from build123d import *

# Parameters (mm, degrees)
SCHIZZO1_R                        = 1.5
ESTRUSIONE_ESTRUSIONE1_DEPTH      = 4.5
ESTRUSIONE_ESTRUSIONE1_DEPTH_BACK = 4.5
SCHIZZO2_W                        = 32
SCHIZZO2_H                        = 3
SCHIZZO2_W_2                      = 10
TAGLIO_ESTRUSIONE1_DEPTH          = 12.277661417
TAGLIO_ESTRUSIONE1_DEPTH_BACK     = 23.284267349
TAGLIO_ESTRUSIONE3_DEPTH          = 3.5
RACCORDO1_R                       = 5
RACCORDO2_R                       = 5
RACCORDO3_R                       = 2.5
RACCORDO4_R                       = 2.5


with BuildPart() as part:
    # Schizzo1 → Estrusione-Estrusione1 (new body, two sides)
    with BuildSketch(Plane.XY) as estrusione_estrusione1_sk:
        with BuildLine():
            ThreePointArc((9.895231175, 3), (-10.34, 0), (9.895231175, -3))
            Line((9.895231175, -3), (35, -3))
            ThreePointArc((35, -3), (38, 0), (35, 3))
            Line((35, 3), (9.895231175, 3))
        make_face()
        Circle(SCHIZZO1_R, mode=Mode.SUBTRACT)
        with Locations((35, 0)):
            Circle(SCHIZZO1_R, mode=Mode.SUBTRACT)
    extrude(amount=ESTRUSIONE_ESTRUSIONE1_DEPTH)
    extrude(estrusione_estrusione1_sk.sketch, amount=-ESTRUSIONE_ESTRUSIONE1_DEPTH_BACK)

    # Schizzo2 → Taglio-Estrusione1 (cut, two sides)
    with BuildSketch(Plane(origin=(0, -3, 0), x_dir=(-1, 0, 0), z_dir=(0, -1, 0))) as taglio_estrusione1_sk:
        with Locations((-5.66, 0)):
            Rectangle(SCHIZZO2_W, SCHIZZO2_H)
        with Locations((-33, 0)):
            Rectangle(SCHIZZO2_W_2, SCHIZZO2_H)
    extrude(amount=TAGLIO_ESTRUSIONE1_DEPTH, mode=Mode.SUBTRACT)
    extrude(taglio_estrusione1_sk.sketch, amount=-TAGLIO_ESTRUSIONE1_DEPTH_BACK, mode=Mode.SUBTRACT)

    # Schizzo18 → Taglio-Estrusione3 (cut)
    with BuildSketch(Plane(origin=(0, 0, -4.5), x_dir=(-1, 0, 0), z_dir=(0, 0, -1))):
        with BuildLine():
            Line((-9.895231175, 3), (-5.58530214, 3))
            ThreePointArc((-5.58530214, 3), (6.34, 0), (-5.58530214, -3))
            Line((-5.58530214, -3), (-9.895231175, -3))
            ThreePointArc((-9.895231175, -3), (10.34, 0), (-9.895231175, 3))
        make_face()
    extrude(amount=-TAGLIO_ESTRUSIONE3_DEPTH, mode=Mode.SUBTRACT)

    # Raccordo1
    raccordo1_edges = [part.edges().sort_by_distance(p)[0] for p in [
        (9.895231175, 3, 3),
    ]]
    fillet(raccordo1_edges, radius=RACCORDO1_R)

    # Raccordo2
    raccordo2_edges = [part.edges().sort_by_distance(p)[0] for p in [
        (9.895231175, -3, 3),
    ]]
    fillet(raccordo2_edges, radius=RACCORDO2_R)

    # Raccordo3
    raccordo3_edges = [part.edges().sort_by_distance(p)[0] for p in [
        (5.58530214, 3, -3),
    ]]
    fillet(raccordo3_edges, radius=RACCORDO3_R)

    # Raccordo4
    raccordo4_edges = [part.edges().sort_by_distance(p)[0] for p in [
        (5.58530214, -3, -3),
    ]]
    fillet(raccordo4_edges, radius=RACCORDO4_R)


solid = part.part
Model file for the job. Use its own axes, mm. A direction names the side the tool comes from. Round coordinates to 2 decimals unless told otherwise and drop trailing zeros. Loops run counter-clockwise (first coordinate to the right, second up) from the corner with the lowest first, then second, coordinate; pieces in that order, holes last. Notation, with made-up numbers: M 65,85.25 L 78,85.25 A23 cw 78,96.25 Z; hole C 41.25,-25 d1. An arc over 180 degrees is marked long. One line per question, with ' | ' between items.
1) Mould opens along Z. For faces 5 (the cylindrical face through (5.82, -3.255, -2.979)), 6 (the flat face through (32, 0, 1.5)), 7 (the flat face through (8, 0, 4.5)) say: +Z half, -Z half, draft (parallel to the pull), parting line (faces both ways), or undercut.
Solved:
face 5: draft | face 6: undercut | face 7: +Z half
2) Band-saw the part on C-C (y = 0). Give the cut face in (x, z).
Solved:
outline: M -10.34,1.5 L -1.5,1.5 L -1.5,4.5 L -10.34,4.5 Z; M -6.34,-4.5 L -1.5,-4.5 L -1.5,-1.5 L -6.34,-1.5 Z; M 1.5,-4.5 L 33.5,-4.5 L 33.5,-1.5 L 28,-1.5 L 28,1.5 L 33.5,1.5 L 33.5,4.5 L 1.5,4.5 L 1.5,1.5 L 21.66,1.5 L 21.66,-1.5 L 1.5,-1.5 Z; M 36.5,-4.5 L 38,-4.5 L 38,-1.5 L 36.5,-1.5 Z; M 36.5,1.5 L 38,1.5 L 38,4.5 L 36.5,4.5 Z
3) Drill centre lines: line 1 along X through (y, z) = (0, 2.55); line 2 along X through (y, z) = (0, -3.55); line 3 along Y through (x, z) = (35, -2.4). Where is each one in solid material? Low to high.
Solved:
line 1: x = -10.34 to -1.5, 1.5 to 33.5, 36.5 to 38 | line 2: x = -6.34 to -1.5, 1.5 to 33.5, 36.5 to 38 | line 3: y = -3 to -1.5, 1.5 to 3
4) Band-saw the part on A-A (x = 0). Give the cut face in (y, z).
Solved:
outline: M -10.34,1.5 L -1.5,1.5 L -1.5,4.5 L -10.34,4.5 Z; M -6.34,-4.5 L -1.5,-4.5 L -1.5,-1.5 L -6.34,-1.5 Z; M 1.5,-4.5 L 6.34,-4.5 L 6.34,-1.5 L 1.5,-1.5 Z; M 1.5,1.5 L 10.34,1.5 L 10.34,4.5 L 1.5,4.5 Z
5) 3-axis set-ups, long thin cutter, end or side, ignore diameter. For faces 1 (the cylindrical face through (-6.336, 0.219, -3.021)), 2 (the flat face through (28, 0, 0)), 3 (the flat face through (21.66, 0, 0)), 4 (the cylindrical face through (5.85, 3.24, -2.98)): which of +Z, -Z, +X, -X, +Y, -Y reach the whole face in a straight line?
Solved:
face 1: -Z | face 2: +X, +Y, -Y | face 3: -X, +Y, -Y | face 4: -Z, +X, +Y
6) Band-saw the part on D-D (x = 9.5). Give the cut face in (y, z).
Solved:
outline: M -4.52,1.5 L 4.52,1.5 L 4.52,4.5 L -4.52,4.5 Z; M -3,-4.5 L 3,-4.5 L 3,-1.5 L -3,-1.5 Z
7) Flat gauge pins, fed straight in: pin 1 (2 mm diameter, centred on y = 5, z = -1, fed in from -X); pin 2 (4 mm diameter, centred on x = 21.5, z = -2.5, fed in from +Y); pin 3 (3 mm diameter, centred on x = 1.5, z = -2.5, fed in from -Y). Where does each tip first touch, or does it go through?
Solved:
pin 1: stops at x = -4.81 | pin 2: stops at y = 3 | pin 3: stops at y = -6.34
8) Band-saw the part on B-B (z = -3). Give the cut face in (x, y), then the cut area to 3 significant figures.
Solved:
outline: M 4.96,-3.94 A2.5 cw 6.92,-3 L 35,-3 A3 ccw 35,3 L 6.92,3 A2.5 cw 4.96,3.94 A6.34 ccw long Z; hole C 0,0 d3; hole C 35,0 d3 | area: 300 mm²
